Could you check a few things on this model? Use its own coordinates, in mm. Face numbers are marked on the shaded views. A direction names the side the tool comes from. Give positions to 0.01 mm unless a question says otherwise; leave off trailing zeros. Loops run counter-clockwise (first coordinate to the right, second up) from the corner with the lowest first, then second, coordinate; pieces in that order, holes last. Notation, with made-up numbers: M 26,69.25 L 42,69.25 A25 cw 42,92.25 Z; hole C 58.5,49.25 d7. An arc over 180 degrees is marked long. Use a Markdown table: item, result. Add a question column.
1) If I drill on line 1 along Z through (x, y) = (0, 1.2) (3 decimals); line 2 along Y through (x, z) = (-3.25, 2) (3 decimals), over which ranges is the centre line in solid material (lowest first)? Write a range as [from, to].
2) Will these pins go through, and if not, where does the flat tip stop? pin 1 Ø2 at (y, z) = (4.5, -2.5) entering from -X; pin 2 Ø1 at (y, z) = (-3.5, 5) entering from +X; pin 3 Ø2 at (y, z) = (-4, -3) entering from -X.
3) Suppose I cut it at A-A on z = 0. List the corners of the cut face in (x, y) for me (3 decimals).
4) We'd pull the mould along Z, two halves only. Please class the marked faces 5, 6 and 7: +Z half, -Z half, draft (parallel to the pull), parting line (faces both ways), or undercut.
5) Suppose I cut it at C-C on y = 0.5. List the corners of the cut face in (x, z) for me (3 decimals).
6) Which directions (+Z, -Z, +X, -X, +Y, -Y) give clear straight access to the entire face, cutting with the end or side of a thin tool? Please do the marked faces 1, 2, 3 and 4.
7) Suppose I cut it at B-B on x = 0. List the corners of the cut face in (y, z) for me (3 decimals), and give its area (3 significant figures).
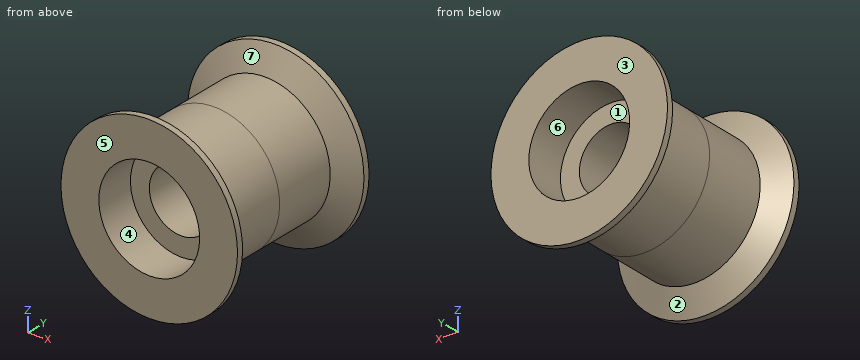
```python
from build123d import *


with BuildPart() as part:
    # Sketch2 → Revolve1 (revolve)
    with BuildSketch(Plane(origin=(0, 0, 0), x_dir=(0, 0, -1), z_dir=(1, 0, 0))):
        Polygon((2.5, 0), (2.5, 3.375), (4, 3.375), (4, 6.5), (7, 6.5), (7, 6), (5.125, 5), (5.125, 0), align=None)
    revolve1 = revolve(axis=Axis((0, 0, 0), (0, 1, 0)))

    # Mirror1: Revolve1 across plane
    add(revolve1.mirror(Plane.ZX))


solid = part.part
```
Answer block:
| question | item | result |
|---|---|---|
| 1 | line 1 | z = [-5.125, -2.5], [2.5, 5.125] |
| 1 | line 2 | y = [-3.375, 3.375] |
| 2 | pin 1 | stops at x = -5.57 |
| 2 | pin 2 | stops at x = 2.45 |
| 2 | pin 3 | stops at x = -4.72 |
| 3 | outline | M -7,-6.5 L -4,-6.5 L -4,-3.375 L -2.5,-3.375 L -2.5,3.375 L -4,3.375 L -4,6.5 L -7,6.5 L -7,6 L -5.125,5 L -5.125,-5 L -7,-6 Z; M 2.5,-3.375 L 4,-3.375 L 4,-6.5 L 7,-6.5 L 7,-6 L 5.125,-5 L 5.125,5 L 7,6 L 7,6.5 L 4,6.5 L 4,3.375 L 2.5,3.375 Z |
| 4 | face 5 | draft |
| 4 | face 6 | undercut |
| 4 | face 7 | parting line |
| 5 | outline | C 0,0 d10.25; hole C 0,0 d5 |
| 6 | face 1 | +Y |
| 6 | face 2 | none |
| 6 | face 3 | +Z, -Z, +X, -X, +Y |
| 6 | face 4 | -Y |
| 7 | outline | M -6.5,-7 L -6,-7 L -5,-5.125 L 5,-5.125 L 6,-7 L 6.5,-7 L 6.5,-4 L 3.375,-4 L 3.375,-2.5 L -3.375,-2.5 L -3.375,-4 L -6.5,-4 Z; M -6.5,4 L -3.375,4 L -3.375,2.5 L 3.375,2.5 L 3.375,4 L 6.5,4 L 6.5,7 L 6,7 L 5,5.125 L -5,5.125 L -6,7 L -6.5,7 Z |
| 7 | area | 57.0 mm^2 |
